Model file for the job. Use its own axes, mm. Face numbers are marked on the shaded views. A direction names the side the tool comes from. Round coordinates to 2 decimals unless told otherwise and drop trailing zeros. Order: outer loops, then holes, each group sorted by start corner. A loop starts at its lowest first (then second) coordinate and runs counter-clockwise, first axis right, second up. Notation, with made-up numbers: (81, 80.5) -> (93, 80.5) arc R22 cw to (93, 91.5) -> close; hole circle Ø5 at (-14, 20.5). An arc over 180 degrees is marked (long way). Put each result on its own line as item: value. Start each with the question number.
Q1. Pull direction X, two halves, no side cores. Call the marked faces 4, 5 and 6: released by +X, released by -X, zero draft, split by the parting line, or undercut.
Q2. Cut at C-C, the plane z = 23. List the corners of the cut face in (x, y), and give its area (3 significant figures).
Q3. 3-axis set-ups, long thin cutter, end or side, ignore diameter. For the marked faces 1, 2 and 3: which of +Z, -Z, +X, -X, +Y, -Y reach the whole face in a straight line?
Q4. Cut at D-D, the plane x = 1. List the corners of the cut face in (y, z) (3 decimals), and give its area (3 significant figures).
Q5. Flat gauge pins, fed straight in: P1, Ø12, axis at x = -22.5, y = 17, coming from the -Z side; P2, Ø8, axis at x = -39, z = 47.5, coming from the +Y side (3 decimals); P3, Ø9, axis at x = -16, z = 12.5, coming from the -Y side; P4, Ø2.5, axis at x = -44.5, y = 77.5, coming from the +Z side. Where does each tip first touch, or does it go through?
Q6. Cut at A-A, the plane z = 31. List the corners of the cut face in (x, y).
Q7. Probe L1, parallel to X at y = 96.5, z = 19; L2, parallel to Z at x = -9.5, y = 7; L3, parallel to Y at x = 3.5, z = -1. List the from-to ranges inside material, lowest first.
Q8. Cut at B-B, the plane z = 50. List the corners of the cut face in (x, y) (3 decimals), and give its area (3 significant figures).
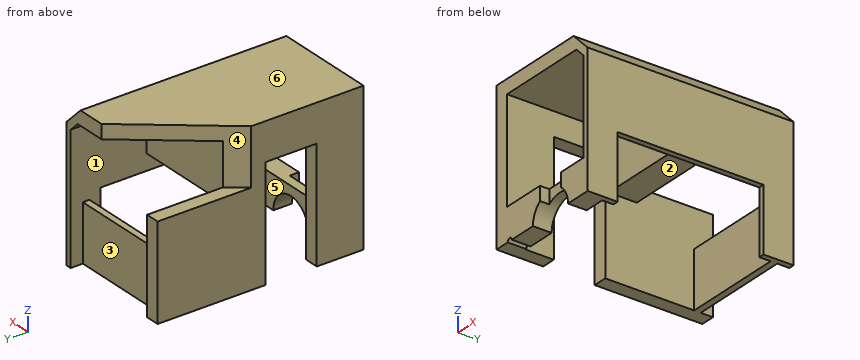
Autodesk Inventor part; units mm, degrees
ref_plane "YZ Plane" through (0, 0, 0) normal (1, 0, 0) x (0, 1, 0)
ref_plane "XZ Plane" through (0, 0, 0) normal (0, 1, 0) x (-1, 0, 0)
ref_plane "XY Plane" through (0, 0, 0) normal (0, 0, 1) x (1, 0, 0)
sketch "Sketch1" plane through (0, 0, 0) normal (0, 1, 0) x (-1, 0, 0)
  line L0 (48.2977, 71.5211) -> (-16.7023, 71.5211)
  line L1 (-16.7023, 71.5211) -> (-16.7023, -8.4789)
  line L2 (-16.7023, -8.4789) -> (48.2977, -8.4789)
  line L3 (48.2977, -8.4789) -> (48.2977, 71.5211)
  arc A0 (22.2975, -8.4789) -> (-2.7023, -8.4789) centre (9.7976, -8.4281) ccw
  line L4 (-16.7023, -8.4789) -> (-13.7023, -8.4789)
  line L5 (-13.7023, -8.4789) -> (-13.7023, 71.5211)
  line L6 (-13.7023, 71.5211) -> (-16.7023, 71.5211)
  line L7 (-16.7023, 71.5211) -> (-16.7023, -8.4789)
  line L8 (48.2977, -8.4789) -> (40.7977, -8.4789)
  line L9 (40.7977, -8.4789) -> (40.7977, 71.5211)
  line L10 (40.7977, 71.5211) -> (48.2977, 71.5211)
  line L11 (48.2977, 71.5211) -> (48.2977, -8.4789)
  line L12 (-13.7023, -8.4789) -> (40.7977, -8.4789)
  line L13 (40.7977, -8.4789) -> (40.7977, 9.0211)
  line L14 (40.7977, 9.0211) -> (-13.7023, 9.0211)
  line L15 (-13.7023, 9.0211) -> (-13.7023, -8.4789)
  line L16 (-13.7023, 71.5211) -> (40.7977, 71.5211)
  line L17 (40.7977, 71.5211) -> (40.7977, 64.0211)
  line L18 (40.7977, 64.0211) -> (-13.7023, 64.0211)
  line L19 (-13.7023, 64.0211) -> (-13.7023, 71.5211)
  line L20 (-16.7023, 61.5211) -> (-6.7023, 71.5211)
  line L21 (-16.7023, 61.5211) -> (-16.7023, 71.5211)
  line L22 (-6.7023, 71.5211) -> (-13.7023, 64.5211)
  line L23 (-13.7023, 64.0211) -> (-13.7023, 64.5211)
  line L24 (-6.7023, 71.5211) -> (40.7977, 71.5211)
  line L25 (40.7977, 64.0211) -> (-13.7023, 64.0211)
  line L26 (-13.7023, 64.5211) -> (-13.7023, 64.0211)
  line L27 (-13.7023, 64.5211) -> (-6.7023, 71.5211)
  line L28 (-13.7023, 54.0211) -> (-3.7023, 64.0211)
  point P0 (0, 0)
  dimension "d0" = 80
  dimension "d1" = 65
  dimension "d3" = 14
  dimension "d4" = 12.5
  dimension "d5" = 7.5
  dimension "d6" = 3
  dimension "d7" = 17.5
  dimension "d8" = 7.5
  dimension "d9" = 10
  dimension "d10" = 10
  dimension "d48" = 10
  dimension "d49" = 10
extrude "Extrusion1" add sketch "Sketch1" along normal blind 110 contours L3 L2 L9 L0 | L9 L18 L5 L20 L0 | L2 A0 L5 L14 L9 | L5 L2 L1 L20
sketch "Sketch2" plane through (-22.2975, 0, -8.4789) normal (0, 0, -1) x (-1, 0, 0)
  line L0 (18.5002, 0) -> (18.5002, 110)
  line L1 (18.5002, 110) -> (-35.9998, 110)
  line L2 (-35.9998, 110) -> (-35.9998, 10)
  line L3 (-35.9998, 10) -> (18.5002, 10)
  line L4 (18.5002, 10) -> (18.5002, 110)
  point P0 (-22.2975, 0)
  dimension "d13" = 100
  dimension "d14" = 54.5
extrude "Extrusion2" cut sketch "Sketch2" against normal blind 30
sketch "Sketch3" plane through (-40.7977, 0, 9.0211) normal (0, 0, 1) x (1, 0, 0)
  line L0 (54.5, 10) -> (0, 10)
  line L1 (26.0002, 10) -> (36, 10)
  line L2 (18.5002, 10) -> (18.5002, 0)
  line L3 (43.5, 0) -> (43.5, 10)
  line L4 (0, 0) -> (54.5, 0)
  line L5 (38.5, 0) -> (23.5002, 0)
  line L6 (23.5002, 0) -> (23.5002, 5)
  line L7 (23.5002, 5) -> (38.5, 5)
  line L8 (38.5, 5) -> (38.5, 0)
  point P0 (40.7977, 0)
  dimension "d43" = 5
  dimension "d44" = 5
  dimension "d45" = 5
sketch "Sketch4" plane through (16.7023, 0, 61.5211) normal (1, 0, 0) x (0, 0, -1)
  line L0 (70, 110) -> (70, 10)
  line L1 (70, 94) -> (36, 94)
  line L2 (36, 94) -> (36, 16)
  line L3 (36, 16) -> (70, 16)
  line L4 (70, 16) -> (70, 94)
  line L5 (0, 0) -> (70, 0)
  line L6 (0, 110) -> (70, 110)
  point P0 (61.5211, 0)
  dimension "d22" = 34
  dimension "d23" = 16
  dimension "d24" = 16
  dimension "d25" = 78
extrude "Extrusion4" cut sketch "Sketch4" against normal blind 30
sketch "Sketch5" plane through (0, 0, 0) normal (0, -1, 0) x (1, 0, 0)
  line L0 (-40.7977, -8.4789) -> (-22.2975, -8.4789)
  arc A0 (-40.2975, -8.4789) -> (-37.2975, -8.4789) centre (-38.7975, -8.4789) ccw
  arc A1 (-37.2975, -8.4789) -> (-40.2975, -8.4789) centre (-38.7975, -8.4789) ccw
  point P0 (0, 0)
  dimension "d28" = 18
  dimension "d29" = 1.5
  dimension "d30" = 0
  dimension "d31" = 1.5
extrude "Extrusion5" cut sketch "Sketch5" against normal blind 30 contours A1 L0
sketch "Sketch7" plane through (-48.2977, 0, 71.5211) normal (0, 0, 1) x (1, 0, 0)
  line L0 (0, 110) -> (55, 110)
  line L1 (0, 110) -> (40, 110)
  line L2 (40, 110) -> (0, 60)
  line L3 (0, 60) -> (0, 110)
  line L4 (65, 110) -> (65, 0)
  point P0 (48.2977, 0)
  dimension "d39" = 40
  dimension "d40" = 25
  dimension "d41" = 50
extrude "Extrusion6" cut sketch "Sketch3" against normal blind 30 contours L4 L6 L7 L8
sketch "Sketch8" plane through (0, 110, 0) normal (0, 1, 0) x (1, 0, 0)
  line L0 (13.7023, 8.4789) -> (13.7023, -64.0211)
  line L1 (13.7023, -59.0211) -> (8.7023, -64.0211)
  line L2 (8.7023, -64.0211) -> (13.7023, -64.0211)
  line L3 (13.7023, -64.0211) -> (13.7023, -59.0211)
  point P0 (0, 0)
  dimension "d50" = 5
  dimension "d51" = 5
extrude "Extrusion7" add sketch "Sketch8" against normal up to surface (110 mm away)
extrude "Extrusion8" cut sketch "Sketch7" against normal blind 30
sketch "Sketch9" plane through (13.7023, 0, 9.0211) normal (-1, 0, 0) x (0, 0, 1)
  line L0 (32.5, 69.375) -> (55, 69.375)
  line L1 (50, 0) -> (50, 110)
  line L2 (50, 69.375) -> (25, 69.375)
  line L3 (25, 69.375) -> (25, 54.375)
  line L4 (25, 54.375) -> (50, 54.375)
  line L5 (50, 54.375) -> (50, 69.375)
  point P0 (-9.0211, 0)
  dimension "d56" = 15
  dimension "d57" = 25
extrude "Extrusion9" add sketch "Sketch9" along normal up to next
sketch "Sketch10" plane through (-40.7977, 54.375, 59.0211) normal (0, 0, 1) x (1, 0, 0)
  line L0 (54.5, 15) -> (0, 15)
  line L1 (55.1529, 0) -> (0.519, 0)
  line L2 (0.519, 0) -> (0.519, 15)
  line L3 (0.519, 15) -> (55.1529, 15)
  line L4 (55.1529, 15) -> (55.1529, 0)
  line L5 (54.5, 0) -> (0, 0)
  line L6 (0, 15) -> (27.836, 15)
  line L7 (27.836, 15) -> (27.836, 0)
  line L8 (27.836, 0) -> (0, 0)
  line L9 (0, 0) -> (0, 15)
  point P0 (40.7977, -54.375)
extrude "Extrusion10" add sketch "Sketch10" along normal up to next
sketch "Sketch11" plane through (13.7023, 0, 9.0211) normal (-1, 0, 0) x (0, 0, 1)
  line L0 (-17.5, 94) -> (-17.5, 110)
  line L1 (-17.5, 100) -> (12.5, 100)
  line L2 (12.5, 100) -> (12.5, 103.5)
  line L3 (12.5, 103.5) -> (-17.5, 103.5)
  line L4 (-17.5, 103.5) -> (-17.5, 100)
  line L5 (-17.5, 110) -> (50, 110)
  point P0 (-9.0211, 0)
  dimension "d62" = 3.5
  dimension "d63" = 30
  dimension "d64" = 10
extrude "Extrusion11" add sketch "Sketch11" along normal up to next
sketch "Sketch12" plane through (-48.2977, 0, -8.4789) normal (-1, 0, 0) x (0, 0, 1)
  line L0 (0, 100) -> (0, 10)
  line L1 (0, 52.5) -> (60, 52.5)
  line L2 (60, 52.5) -> (60, 25)
  line L3 (60, 25) -> (0, 25)
  line L4 (0, 25) -> (0, 52.5)
  line L5 (80, 0) -> (80, 60)
  line L6 (80, 60) -> (50, 60)
  point P0 (8.4789, 0)
  dimension "d67" = 27.5
  dimension "d68" = 60
  dimension "d69" = 20
  dimension "d70" = 7.5
extrude "Extrusion12" cut sketch "Sketch12" against normal up to surface (62 mm away)
equation "\"d8\" = d5"
equation "\"d49\" = d48"
equation "\"d44\" = d43"
equation "\"d24\" = d23"
equation "\"d31\" = d29"
equation "\"d50\" = d51"
properties part number "Basev3.2"
Ans:
1. face 4: released by -X
1. face 5: undercut
1. face 6: zero draft
2. outline: (-48.3, 0) -> (-40.8, 0) -> (-40.8, 25) -> (-48.3, 25) -> close; (-48.3, 52.5) -> (-40.8, 52.5) -> (-40.8, 110) -> (-48.3, 110) -> close; (13.7, 0) -> (16.7, 0) -> (16.7, 16) -> (13.7, 16) -> close; (13.7, 94) -> (16.7, 94) -> (16.7, 110) -> (13.7, 110) -> close
2. area: 715 mm^2
3. face 1: none
3. face 2: -Z, +Y, -Y
3. face 3: -Z, +Y
4. outline: (0, -2.13) -> (10, -2.13) -> (10, 9.021) -> (0, 9.021) -> close; (0, 64.021) -> (54.375, 64.021) -> (54.375, 34.021) -> (69.375, 34.021) -> (69.375, 64.021) -> (110, 64.021) -> (110, 71.521) -> (0, 71.521) -> close; (100, -8.479) -> (103.5, -8.479) -> (103.5, 21.521) -> (100, 21.521) -> close
4. area: 1,490 mm^2
5. P1: stops at z = 64.02
5. P2: stops at y = 69.375
5. P3: stops at y = 0
5. P4: stops at z = 41.52
6. outline: (-48.3, 0) -> (-40.8, 0) -> (-40.8, 25) -> (-48.3, 25) -> close; (-48.3, 52.5) -> (-40.8, 52.5) -> (-40.8, 110) -> (-48.3, 110) -> close; (13.7, 0) -> (16.7, 0) -> (16.7, 110) -> (13.7, 110) -> close
7. L1: x = -48.3 to -40.8, 13.7 to 16.7
7. L2: z = 4.07 to 9.02, 64.02 to 71.52
7. L3: y = 0 to 10, 100 to 103.5
8. outline: (-48.298, 0) -> (-40.798, 0) -> (-40.798, 25) -> (-48.298, 25) -> close; (-48.298, 52.5) -> (-40.798, 52.5) -> (-40.798, 54.375) -> (13.702, 54.375) -> (13.702, 0) -> (16.702, 0) -> (16.702, 110) -> (13.702, 110) -> (13.702, 69.375) -> (-40.798, 69.375) -> (-48.298, 60) -> close
8. area: 1,430 mm^2
